Geometry check sheet. Reference: the model listing, model coordinates, mm. A direction names the side the tool comes from. Round coordinates to 2 decimals unless told otherwise and drop trailing zeros. Loops run counter-clockwise (first coordinate to the right, second up) from the corner with the lowest first, then second, coordinate; pieces in that order, holes last. Notation, with made-up numbers: M 44,-6.75 L 92,-6.75 A34 ccw 92,28.25 Z; hole C -12.75,13.25 d8. An arc over 180 degrees is marked long. Answer in a Markdown table with one row per item. Add a question column.
Autodesk Inventor part; units mm, degrees
ref_plane "YZ Plane" through (0, 0, 0) normal (1, 0, 0) x (0, 1, 0)
ref_plane "XZ Plane" through (0, 0, 0) normal (0, 1, 0) x (-1, 0, 0)
ref_plane "XY Plane" through (0, 0, 0) normal (0, 0, 1) x (1, 0, 0)
sketch "Sketch3" plane through (0, 0, 0) normal (1, 0, 0) x (0, 1, 0)
  circle A0 centre (0, 0) radius 1.5
  arc A1 (1.725, -2.4545) -> (-1.6531, -2.5034) centre (0, 0) ccw
  line L0 (-0.7552, -4.1724) -> (-0.7552, -10)
  line L1 (-0.7552, -10) -> (0.875, -10)
  line L2 (0.875, -10) -> (0.875, -4.0908)
  arc A2 (1.725, -2.4545) -> (0.875, -4.0908) centre (2.875, -4.0908) ccw
  arc A3 (-0.7552, -4.1724) -> (-1.6531, -2.5034) centre (-2.7552, -4.1724) ccw
  dimension "d4" = 3
  dimension "d5" = 6
  dimension "d7" = 2
extrude "Extrusion2" add sketch "Sketch3" along normal blind 30
chamfer "Chamfer1" distance 0.25 angle 45 16 edges at (30, 0.875, -7.0454) (30, 1.1002, -3.1688) (30, -0.0435, 2.9997) (30, -0.9939, -3.2248) (30, -0.7552, -7.0862) (30, 0.0599, -10) (30, -1.5, 0) (0, -1.5, 0) (0, -0.0435, 2.9997) (0, -0.9939, -3.2248) (0, -0.7552, -7.0862) (0, 1.1002, -3.1688) (0, 0.875, -7.0454) (0, 0.0599, -10) (15, 0.875, -10) (15, -0.7552, -10)
properties part number "CoinLock"
1) Thickness scan on L1, parallel to Z at x = 22, y = 0; L2, parallel to Y at x = 18, z = -0.75; L3, parallel to Y at x = 4.5, z = -7 (3 decimals). Record the ranges inside material, lowest first. Write a range as [from, to].
2) Cross-section at B-B, the plane z = -6.25. Record the boundary of the cut face in (x, y) (3 decimals), plus the area to 3 significant figures.
3) Set-up check for faces 5 (the flat face through (0, 0, -2)), 6 (the flat face through (15, 0.875, -7)), 7 (the flat face through (15, -0.755, -7)): record each of +Z, -Z, +X, -X, +Y, -Y from which the full face is reachable in a straight line by a thin tool's end or side.
4) Go/stop test with flat-tipped pins: pin 1 (6 mm diameter, centred on x = 14.5, z = -6.5, fed in from +Y); pin 2 (3 mm diameter, centred on x = 21.5, z = -7, fed in from -Y). Record where each tip stops, or that it passes through.
5) Draft check along Z on faces 1 (the cylindrical face through (14.794, 1.094, -3.181)), 2 (the cylindrical face through (15, 0, 3)), 3 (the flat face through (30, 0, -2)), 4 (the cylindrical face through (14.79, -1.5, -0.07)). Enter one of: +Z half, -Z half, draft (parallel to the pull), parting line (faces both ways), or undercut.
Worked answers:
| question | item | result |
|---|---|---|
| 1 | L1 | z = [-10, -1.5], [1.5, 3] |
| 1 | L2 | y = [-2.9, -1.3], [1.3, 2.9] |
| 1 | L3 | y = [-0.755, 0.875] |
| 2 | outline | M 0,-0.505 L 0.25,-0.755 L 29.75,-0.755 L 30,-0.505 L 30,0.625 L 29.75,0.875 L 0.25,0.875 L 0,0.625 Z |
| 2 | area | 48.8 mm2 |
| 3 | face 5 | +Z, -Z, -X, +Y, -Y |
| 3 | face 6 | -Z, +X, -X, +Y |
| 3 | face 7 | -Z, +X, -X, -Y |
| 4 | pin 1 | stops at y = 0.96 |
| 4 | pin 2 | stops at y = -0.76 |
| 5 | face 1 | -Z half |
| 5 | face 2 | parting line |
| 5 | face 3 | draft |
| 5 | face 4 | undercut |
